Build history of the part. All positions in model axes, mm. Face numbers are marked on the shaded views. A direction names the side the tool comes from. Give positions to 0.01 mm unless a question says otherwise; leave off trailing zeros. Order: outer loops, then holes, each group sorted by start corner. A loop starts at its lowest first (then second) coordinate and runs counter-clockwise, first axis right, second up. Notation, with made-up numbers: (60, 7.25) -> (118, 7.25) arc R28 cw to (118, 43.25) -> close; hole circle Ø11 at (32.25, 81). An arc over 180 degrees is marked (long way). One line per question, with ' | ' between items. Start each with the question number.
(1) Cut at C-C (z = 12). Give the number of separate pieces and of enclosed holes in the cut face, then the cut area to 3 significant figures.
(2) Cut at A-A (x = -22). Give the cut face in (y, z), then the cut area to 3 significant figures.
(3) Drill centre lines: L1, parallel to Y at x = -69, z = 38; L2, parallel to Y at x = -64.5, z = 12; L3, parallel to X at y = -8, z = 14.5. Where is each one in solid material? Low to high. Write a range as from..to.
(4) Which spindle directions (+Z, -Z, +X, -X, +Y, -Y) get a long thin tool onto all of the face, cutting with end or side? Do the marked faces 4, 5, 6, 7 and 8. Say none if no direction does.
(5) Pull direction X, two halves, no side cores. Call the marked faces 1, 2 and 3: +X half, -X half, draft (parallel to the pull), parting line (faces both ways), or undercut.
(6) Pin check, flat tips, straight feed: pin 1 Ø3 at (y, z) = (14, 35) entering from -X; pin 2 Ø3.5 at (x, z) = (-63.88, 26.5) entering from -Y; pin 3 Ø12 at (x, z) = (-53.5, 43) entering from +Y; pin 4 Ø4 at (x, z) = (-64, 25.5) entering from -Y. Stop position of each tip, or through.
Solid Edge part; units mm, degrees
sketch "Sketch1" plane through (0, 0, 0) normal (0, 0, 1) x (1, 0, 0)
  line L0 (-50.4769, -0.1262) -> (-31.3427, -46.3202)
  line L1 (-31.3427, -46.3202) -> (-10.2002, -25.1777)
  line L2 (-10.2002, -25.1777) -> (-24.3402, -25.1777)
  line L3 (-24.3402, -25.1777) -> (26.5942, 25.7567)
  line L4 (26.5942, 25.7567) -> (19.5231, 32.8278)
  line L5 (19.5231, 32.8278) -> (-26.4388, -13.1341)
  line L6 (-26.4388, -13.1341) -> (-50.4769, -0.1262)
  dimension "D1" = 50.4769
  dimension "D2" = 31.3427
  dimension "D3" = 26.5942
  dimension "D4" = 19.5231
  dimension "D5" = 10.2002
extrude "Protrusion1" add sketch "Sketch1" along normal blind 35
sketch "Sketch2" plane through (-12.0121, -6.8169, 0) normal (0, 0, -1) x (-0.8794859, 0.4759249, 0)
  line L0 (-1.7996, -43.9425) -> (-10.3318, -15.2857)
  line L1 (-10.3318, -15.2857) -> (2.1041, -22.0153)
  line L2 (2.1041, -22.0153) -> (-18.451, 47.0217)
  line L3 (-18.451, 47.0217) -> (6.4693, 54.4415)
  line L4 (6.4693, 54.4415) -> (28.4484, -19.3779)
  line L5 (28.4484, -19.3779) -> (-1.7996, -43.9425)
extrude "Extrusionsausprägung_6" add sketch "Sketch2" against normal blind 4
sketch "Sketch3" plane through (-3.4579, 9.8468, 19.5) normal (-0.7071068, 0.7071068, 0) x (0, 0, 1)
  circle A0 centre (-6.5, 10.45) radius 3.5
  circle A1 centre (-6.5, -19.55) radius 3.5
  dimension "D1" = 6.5
extrude "Cutout1" cut sketch "Sketch3" against normal through all
sketch "Sketch4" plane through (-11.9413, -6.7462, 35) normal (0, 0, 1) x (0.8794859, -0.4759249, 0)
  line L0 (-37.0421, -12.5178) -> (1.771, -44.0384)
  line L1 (1.771, -44.0384) -> (3.3235, -45.2992)
  line L2 (-40.0351, -68.7623) -> (3.3235, -45.2992)
  line L3 (-63.8314, -24.788) -> (-40.0351, -68.7623)
  line L4 (-38.6875, -11.1816) -> (-63.8314, -24.788)
  line L5 (-37.0421, -12.5178) -> (-38.6875, -11.1816)
  dimension "D1" = 63.8314
  dimension "D2" = 40.0351
  dimension "D3" = 1.771
extrude "Extrusionsausprägung_7" add sketch "Sketch4" against normal blind 37 and the other way blind 13
chamfer "Fase_3" distance 3 angle 45 2 edges at (1.127, 0.2895, 0) (-20.7715, -35.7489, 0)
sketch "Sketch5" plane through (-55.2273, -48.1679, 23) normal (0, -1, 0) x (-1, 0, 0)
  circle A0 centre (8.65, -3.5) radius 1.875
  dimension "D1" = 8.65
  dimension "D2" = 8.65
extrude "Extrusionsausschnitt_6" cut sketch "Sketch5" against normal blind 16
chamfer "Fase_4" distance 0.5 angle 45 1 edges at (-62.0023, -48.1679, 26.5)
sketch "Sketch6" plane through (-79.8773, -23.1679, 23) normal (-1, 0, 0) x (0, 0, 1)
  circle A0 centre (-11, 7.5) radius 2.85
  circle A1 centre (15, -10.5) radius 2.85
  dimension "D1" = 15
extrude "Extrusionsausschnitt_7" cut sketch "Sketch6" against normal blind 30
chamfer "Fase_5" distance 0.8 angle 45 2 edges at (-79.8773, -15.6679, 9.15) (-79.8773, -33.6679, 35.15)
properties material "Nylon, allgemein"
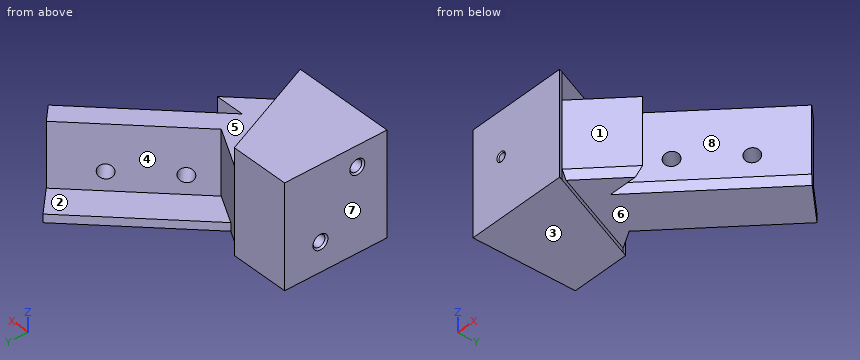
Result set:
1) separate pieces: 3 | enclosed holes: 0 | area: 2,970 mm2
2) outline: (-36.98, 3) -> (-32.73, 0) -> (-25.18, 0) -> (-25.18, 35) -> (-36.98, 35) -> close; (-22.84, 3) -> (-18.59, 0) -> (13.93, 0) -> (13.93, 4) -> (-8.7, 4) -> (-8.7, 35) -> (-22.84, 35) -> close | area: 986 mm2
3) L1: y = -48.17..-36.52, -30.82..1.83 | L2: y = -48.17..-18.52, -12.82..1.83 | L3: x = -79.88..-35.93, -21.3..-17.73, -8.79..-7.16
4) face 4: +Z, +Y | face 5: +Z, +X, +Y | face 6: -Z, +X, +Y | face 7: +Z, -Z, -X, +Y, -Y | face 8: +Z, -Z, +X
5) face 1: +X half | face 2: undercut | face 3: draft
6) pin 1: stops at x = -0.8 | pin 2: stops at y = -32.17 | pin 3: stops at y = 1.83 | pin 4: stops at y = -48.17
